```python
from build123d import *

# Parameters (mm, degrees)
SKETCH1_W               = 50.8
SKETCH1_H               = 50.8
SKETCH1_W_2             = 47.625
SKETCH1_H_2             = 47.625
BOSS_EXTRUDE1_DEPTH     = 304.8
SKETCH6_R               = 2.0955
CUT_EXTRUDE3_DEPTH      = 1
CUT_EXTRUDE3_DEPTH_BACK = 51.8
SKETCH7_R               = 2.0955
CUT_EXTRUDE4_DEPTH      = 1
CUT_EXTRUDE4_DEPTH_BACK = 51.8
SKETCH8_R               = 2.0955
CUT_EXTRUDE5_DEPTH      = 51.8
SKETCH9_R               = 2.0955
CUT_EXTRUDE6_DEPTH      = 51.8
SKETCH10_R              = 3.175
CUT_EXTRUDE7_DEPTH      = 5.08
SKETCH11_R              = 3.175
CUT_EXTRUDE8_DEPTH      = 5.08
SKETCH12_R              = 3.175
CUT_EXTRUDE9_DEPTH      = 5.08
SKETCH13_R              = 3.175
CUT_EXTRUDE10_DEPTH     = 5.08
SKETCH15_R              = 1.778
SKETCH15_R_2            = 3.175
CUT_EXTRUDE12_DEPTH     = 5.08
SKETCH16_R              = 1.778
CUT_EXTRUDE13_DEPTH     = 5.08
SKETCH17_R              = 1.778
CUT_EXTRUDE14_DEPTH     = 5.08
SKETCH19_R              = 1.778
SKETCH19_R_2            = 3.175
CUT_EXTRUDE15_DEPTH     = 5.08


with BuildPart() as part:
    # Sketch1 → Boss-Extrude1 (new body)
    with BuildSketch(Plane(origin=(0, 0, 0), x_dir=(1, 0, 0), z_dir=(0, 1, 0))):
        Rectangle(SKETCH1_W, SKETCH1_H)
        Rectangle(SKETCH1_W_2, SKETCH1_H_2, mode=Mode.SUBTRACT)
    extrude(amount=BOSS_EXTRUDE1_DEPTH)

    # Sketch6 → Cut-Extrude3 (cut, two sides)
    with BuildSketch(Plane(origin=(25.4, 0, 0), x_dir=(0, 0, -1), z_dir=(1, 0, 0))) as cut_extrude3_sk:
        with Locations((0, 12.412400118)):
            Circle(SKETCH6_R)
    extrude(amount=CUT_EXTRUDE3_DEPTH, mode=Mode.SUBTRACT)
    extrude(cut_extrude3_sk.sketch, amount=-CUT_EXTRUDE3_DEPTH_BACK, mode=Mode.SUBTRACT)

    # Sketch7 → Cut-Extrude4 (cut, two sides)
    with BuildSketch(Plane(origin=(0, 0, -25.4), x_dir=(-1, 0, 0), z_dir=(0, 0, -1))) as cut_extrude4_sk:
        with Locations((0, 12.412400118)):
            Circle(SKETCH7_R)
    extrude(amount=CUT_EXTRUDE4_DEPTH, mode=Mode.SUBTRACT)
    extrude(cut_extrude4_sk.sketch, amount=-CUT_EXTRUDE4_DEPTH_BACK, mode=Mode.SUBTRACT)

    # Sketch8 → Cut-Extrude5 (cut, through all)
    with BuildSketch(Plane(origin=(25.4, 0, 0), x_dir=(0, 0, -1), z_dir=(1, 0, 0))):
        with Locations((0, 298.45)):
            Circle(SKETCH8_R)
    extrude(amount=-CUT_EXTRUDE5_DEPTH, mode=Mode.SUBTRACT)

    # Sketch9 → Cut-Extrude6 (cut, through all)
    with BuildSketch(Plane.XY.offset(25.4)):
        with Locations((0, 298.45)):
            Circle(SKETCH9_R)
    extrude(amount=-CUT_EXTRUDE6_DEPTH, mode=Mode.SUBTRACT)

    # Sketch10 → Cut-Extrude7 (cut)
    with BuildSketch(Plane.XY.offset(25.4)):
        with Locations((19.05, 285.75)):
            Circle(SKETCH10_R)
    extrude(amount=-CUT_EXTRUDE7_DEPTH, mode=Mode.SUBTRACT)

    # Sketch11 → Cut-Extrude8 (cut)
    with BuildSketch(Plane.ZY.offset(25.4)):
        with Locations((19.05, 285.75)):
            Circle(SKETCH11_R)
    extrude(amount=-CUT_EXTRUDE8_DEPTH, mode=Mode.SUBTRACT)

    # Sketch12 → Cut-Extrude9 (cut)
    with BuildSketch(Plane(origin=(0, 0, -25.4), x_dir=(-1, 0, 0), z_dir=(0, 0, -1))):
        with Locations((19.05, 285.75)):
            Circle(SKETCH12_R)
    extrude(amount=-CUT_EXTRUDE9_DEPTH, mode=Mode.SUBTRACT)

    # Sketch13 → Cut-Extrude10 (cut)
    with BuildSketch(Plane(origin=(25.4, 0, 0), x_dir=(0, 0, -1), z_dir=(1, 0, 0))):
        with Locations((19.05, 285.75)):
            Circle(SKETCH13_R)
    extrude(amount=-CUT_EXTRUDE10_DEPTH, mode=Mode.SUBTRACT)

    # Sketch15 → Cut-Extrude12 (cut)
    with BuildSketch(Plane(origin=(0, 0, -25.4), x_dir=(-1, 0, 0), z_dir=(0, 0, -1))):
        with Locations((0, 222.25)):
            Circle(SKETCH15_R)
        with Locations((0, 190.5)):
            Circle(SKETCH15_R_2)
    extrude(amount=-CUT_EXTRUDE12_DEPTH, mode=Mode.SUBTRACT)

    # Sketch16 → Cut-Extrude13 (cut)
    with BuildSketch(Plane(origin=(25.4, 0, 0), x_dir=(0, 0, -1), z_dir=(1, 0, 0))):
        with Locations((0, 254)):
            Circle(SKETCH16_R)
    extrude(amount=-CUT_EXTRUDE13_DEPTH, mode=Mode.SUBTRACT)

    # Sketch17 → Cut-Extrude14 (cut)
    with BuildSketch(Plane.ZY.offset(25.4)):
        with Locations((0, 203.2)):
            Circle(SKETCH17_R)
    extrude(amount=-CUT_EXTRUDE14_DEPTH, mode=Mode.SUBTRACT)

    # Sketch19 → Cut-Extrude15 (cut)
    with BuildSketch(Plane.XY.offset(25.4)):
        with Locations((0, 266.7)):
            Circle(SKETCH19_R)
        with Locations((0, 203.2)):
            Circle(SKETCH19_R_2)
    extrude(amount=-CUT_EXTRUDE15_DEPTH, mode=Mode.SUBTRACT)


solid = part.part
```
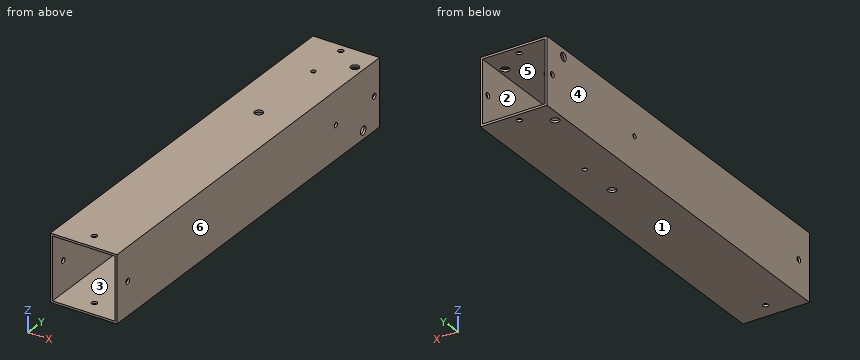
The model under review builds one solid part; all positions refer to its coordinate system, in mm. Face numbers are marked on the shaded views. A direction names the side the tool comes from. Round coordinates to 2 decimals unless told otherwise and drop trailing zeros. Write each loop counter-clockwise with the first axis right and the second up, starting at its lowest first coordinate (ties: lowest second). Pieces come first, ordered by that corner, then holes. Notation, with made-up numbers: (-18, 88.25) - (24, 88.25) arc R22 cw to (24, 94.25) - close; hole circle Ø5 at (2, -33). An arc over 180 degrees is marked (long way). Use one line per item in the form item = value.
Q1. Consider section A-A (z = -19.05). State the section outline as (x, y) points (1 decimal), and give its area (3 significant figures).
Answer key:
outline = (-25.4, 0) - (-23.8, 0) - (-23.8, 304.8) - (-25.4, 304.8) - close; (23.8, 0) - (25.4, 0) - (25.4, 282.6) - (23.8, 282.6) - close; (23.8, 288.9) - (25.4, 288.9) - (25.4, 304.8) - (23.8, 304.8) - close
area = 958 mm2
Q2. Tool access review of the marked faces 5 and 6: name each direction out of +Z, -Z, +X, -X, +Y, -Y from which nothing blocks a thin tool from reaching the whole face with its end or side.
Answer key:
face_5 = +Y, -Y
face_6 = +Z, -Z, +X, +Y, -Y
Q3. Consider section B-B (x = -19.05). State the section outline as (y, z) points (1 decimal), and give its area (3 significant figures).
Answer key:
outline = (0, -25.4) - (282.6, -25.4) - (282.6, -23.8) - (0, -23.8) - close; (0, 23.8) - (304.8, 23.8) - (304.8, 25.4) - (0, 25.4) - close; (288.9, -25.4) - (304.8, -25.4) - (304.8, -23.8) - (288.9, -23.8) - close
area = 958 mm2
Q4. Consider section C-C (y = 274.5). State the section outline as (x, z) points, and give its area (4 significant figures).
Answer key:
outline = (-25.4, -25.4) - (25.4, -25.4) - (25.4, 25.4) - (-25.4, 25.4) - close; hole (-23.81, -23.81) - (23.81, -23.81) - (23.81, 23.81) - (-23.81, 23.81) - close
area = 312.5 mm2
Q5. Consider section D-D (y = 190.5). State the section outline as (x, z) points (1 decimal).
Answer key:
outline = (-25.4, -25.4) - (-3.2, -25.4) - (-3.2, -23.8) - (-23.8, -23.8) - (-23.8, 23.8) - (23.8, 23.8) - (23.8, -23.8) - (3.2, -23.8) - (3.2, -25.4) - (25.4, -25.4) - (25.4, 25.4) - (-25.4, 25.4) - close
Q6. For line 1 (Y direction, x = 0, z = -24.75) (1 decimal); line 2 (X direction, y = 298.45, z = -24.45); line 3 (Z direction, x = -0.5, y = 252), list the stretches that pass through material, from the lowest coordinate up. Write a range as [from, to].
Answer key:
line_1 = [0, 10.3], [14.5, 187.3], [193.7, 220.5], [224, 296.4], [300.5, 304.8]
line_2 = [-25.4, -2.1], [2.1, 25.4]
line_3 = [-25.4, -23.81], [23.81, 25.4]
Q7. Draft analysis for pull direction X (two halves, no side actions). For the marked faces 1, 2, 3 and 4, state which applies: +X half, -X half, draft (parallel to the pull), parting line (faces both ways), or undercut.
Answer key:
face_1 = draft
face_2 = undercut
face_3 = undercut
face_4 = -X half
